```python
from build123d import *

# Parameters (mm, degrees)
SKETCH1_W           = 40.1
SKETCH1_H           = 67.2
SKETCH1_R           = 1.6
BOSS_EXTRUDE1_DEPTH = 2
SKETCH2_W           = 40.1
SKETCH2_H           = 55.2
SKETCH2_W_2         = 25
SKETCH2_H_2         = 2.54
SKETCH2_W_3         = 7.62
BOSS_EXTRUDE2_DEPTH = 3
BOSS_EXTRUDE3_DEPTH = 0.5


with BuildPart() as part:
    # Sketch1 → Boss-Extrude1 (new body)
    with BuildSketch(Plane(origin=(0, 0, 0), x_dir=(0, 0, -1), z_dir=(1, 0, 0))):
        Rectangle(SKETCH1_W, SKETCH1_H)
        with Locations((16.55, 31.1)):
            Circle(SKETCH1_R, mode=Mode.SUBTRACT)
        with Locations((16.55, -31.11)):
            Circle(SKETCH1_R, mode=Mode.SUBTRACT)
        with Locations(Location((-16.55, -31.11, 0), (0, 0, 180))):
            Circle(SKETCH1_R, mode=Mode.SUBTRACT)
        with Locations(Location((-16.55, 31.1, 0), (0, 0, 180))):
            Circle(SKETCH1_R, mode=Mode.SUBTRACT)
    extrude(amount=BOSS_EXTRUDE1_DEPTH)

    # Sketch2 → Boss-Extrude2 (add)
    with BuildSketch(Plane(origin=(2, 0, 0), x_dir=(0, 0, -1), z_dir=(1, 0, 0))):
        with Locations((0, 0.6)):
            Rectangle(SKETCH2_W, SKETCH2_H)
        with Locations((0, -31.6)):
            Rectangle(SKETCH2_W_2, SKETCH2_H_2)
        with Locations((0, 31.6)):
            Rectangle(SKETCH2_W_3, SKETCH2_H_2)
    extrude(amount=BOSS_EXTRUDE2_DEPTH)

    # Sketch3 → Boss-Extrude3 (add)
    with BuildSketch(Plane(origin=(5, 0, 0), x_dir=(0, 0, -1), z_dir=(1, 0, 0))):
        with BuildLine():
            add(Edge.make_bspline(
                [(9.428160808, -10.258647158), (12.148533605, -12.766508078), (15.01174655, -16.60061625), (13.414973779, -29.671171948), (-8.894779227, -22.798689467), (-7.128189514, 1.292467688), (5.124002127, -6.290723583), (9.428160808, -10.258647158)],
                knots=[0, 0, 0, 0, 0.152454057, 0.233716346, 0.541000039, 0.75878804, 1, 1, 1, 1], degree=3))
        make_face()
        with BuildLine():
            add(Edge.make_bspline(
                [(9.428160808, 11.458647158), (12.148533605, 13.966508078), (15.01174655, 17.80061625), (13.414973779, 30.871171948), (-8.894779227, 23.998689467), (-7.128189514, -0.092467688), (5.124002127, 7.490723583), (9.428160808, 11.458647158)],
                knots=[0, 0, 0, 0, 0.152454057, 0.233716346, 0.541000039, 0.75878804, 1, 1, 1, 1], degree=3))
        make_face()
    extrude(amount=BOSS_EXTRUDE3_DEPTH)


solid = part.part
```
Input: part model. Units: mm. Frame: model coordinates. A direction names the side the tool comes from. Round coordinates to 2 decimals unless told otherwise and drop trailing zeros. Loops run counter-clockwise (first coordinate to the right, second up) from the corner with the lowest first, then second, coordinate; pieces in that order, holes last. Notation, with made-up numbers: M -8,87 L 23,87 A22 ccw 23,113 Z; hole C 60.5,-30.75 d4. An arc over 180 degrees is marked long. Answer in a Markdown table with one row per item. Add a question column.
1. Set-up query: faces 1 (the face through (3, 32, 3.81)), 2 (the face through (5, 1, 0)), 3 (the face through (3, -32, -12.5)), 4 (the face through (5, 32, 0)). Return all of +Z, -Z, +X, -X, +Y, -Y with unobstructed straight access to the full face (end or side cutting, diameter ignored); none if empty.
2. Section D-D (z = 9). Output: boundary loops of the cut face in (x, y).
3. Section C-C (x = 2.75). Output: boundary loops of the cut face in (y, z).
4. Mould query, pull axis Y, two halves, no side actions, for faces 5 (the face through (0.99, 32.18, -15.37)), 6 (the face through (0, 0, 0)), 7 (the face through (3, 32.87, 0)), 8 (the face through (1, -33.6, 0)). Classes: released by +Y, released by -Y, zero draft, split by the parting line, or undercut.
5. Section A-A (y = 31.1). Output: boundary loops of the cut face in (x, z), and give its area (3 significant figures).
6. Contact query for flat-ended pins moving along their axis: pin 1 (2 mm diameter, centred on y = 32, z = -2, fed in from +X); pin 2 (3 mm diameter, centred on x = 4, z = 16, fed in from -Y); pin 3 (1.3 mm diameter, centred on x = 3, y = 32, fed in from -Z); pin 4 (2.5 mm diameter, centred on y = -31.11, z = -16.55, fed in from +X) (1 decimal). Output: stop coordinate, or through.
7. Section B-B (z = -16.55). Output: boundary loops of the cut face in (x, y), and give its area (3 significant figures).
8. Ray query, probe 1 along Y at (x, z) = (0.7, 16.55); probe 2 along Y at (x, z) = (2.8, 1); probe 3 along Y at (x, z) = (2.75, -9.5). Return the intervals inside material, ascending.
Values follow:
| question | item | result |
|---|---|---|
| 1 | face 1 | +Z, +X, +Y |
| 1 | face 2 | +X |
| 1 | face 3 | -Z, +X, -Y |
| 1 | face 4 | +Z, -Z, +X, +Y |
| 2 | outline | M 0,-33.6 L 2,-33.6 L 2,-32.87 L 5,-32.87 L 5,-30.33 L 2,-30.33 L 2,-27 L 5,-27 L 5,28.2 L 2,28.2 L 2,33.6 L 0,33.6 Z |
| 3 | outline | M -32.87,-12.5 L -30.33,-12.5 L -30.33,12.5 L -32.87,12.5 Z; M -27,-20.05 L 28.2,-20.05 L 28.2,20.05 L -27,20.05 Z; M 30.33,-3.81 L 32.87,-3.81 L 32.87,3.81 L 30.33,3.81 Z |
| 4 | face 5 | undercut |
| 4 | face 6 | zero draft |
| 4 | face 7 | released by +Y |
| 4 | face 8 | released by -Y |
| 5 | outline | M 0,-20.05 L 2,-20.05 L 2,-18.15 L 0,-18.15 Z; M 0,-14.95 L 2,-14.95 L 2,-3.81 L 5,-3.81 L 5,3.81 L 2,3.81 L 2,14.95 L 0,14.95 Z; M 0,18.15 L 2,18.15 L 2,20.05 L 0,20.05 Z |
| 5 | area | 90.3 mm^2 |
| 6 | pin 1 | x = 5 |
| 6 | pin 2 | y = -27 |
| 6 | pin 3 | z = -3.81 |
| 6 | pin 4 | through |
| 7 | outline | M 0,-33.6 L 2,-33.6 L 2,-32.71 L 0,-32.71 Z; M 0,-29.51 L 2,-29.51 L 2,-27 L 5,-27 L 5,28.2 L 2,28.2 L 2,29.5 L 0,29.5 Z; M 0,32.7 L 2,32.7 L 2,33.6 L 0,33.6 Z |
| 7 | area | 287 mm^2 |
| 8 | probe 1 | -33.6 to -32.71, -29.51 to 29.5, 32.7 to 33.6 |
| 8 | probe 2 | -32.87 to -30.33, -27 to 28.2, 30.33 to 32.87 |
| 8 | probe 3 | -32.87 to -30.33, -27 to 28.2 |
